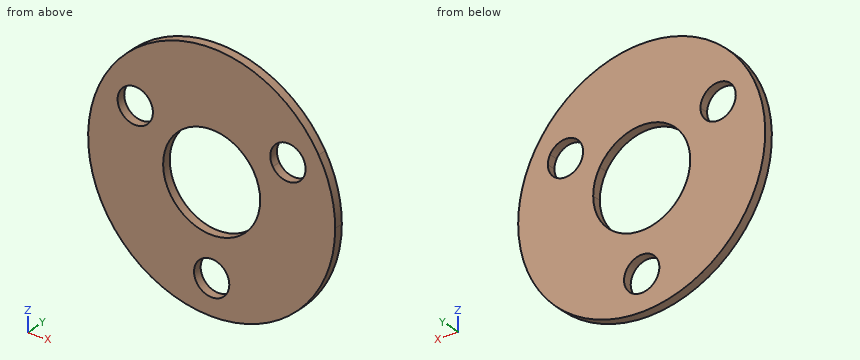
```python
from build123d import *

# Parameters (mm, degrees)
F0_R     = 12.7
F1_DEPTH = 6.35


with BuildPart() as f1:
    # F0 (on Front) → F1 (new body)
    with BuildSketch(Plane.XZ):
        with BuildLine():
            Line((43.995441, 25.40078), (30.245937, 17.4625))
            ThreePointArc((30.245937, 17.4625), (33.734959, 9.039255), (34.925, 0))
            ThreePointArc((34.925, 0), (-9.039255, -33.734959), (-30.245937, 17.4625))
            Line((-30.245937, 17.4625), (-43.994091, 25.4))
            ThreePointArc((-43.994091, 25.4), (-61.342613, 20.751477), (-65.991136, 38.1))
            Line((-65.991136, 38.1), (-76.989658, 44.45))
            ThreePointArc((-76.989658, 44.45), (-23.009013, -85.870806), (88.9, 0))
            ThreePointArc((88.9, 0), (85.870806, 23.009013), (76.989658, 44.45))
            Line((76.989658, 44.45), (65.98911, 38.09883))
            ThreePointArc((65.98911, 38.09883), (67.176599, 35.121917), (67.581014, 31.942516))
            ThreePointArc((67.581014, 31.942516), (58.275364, 19.704527), (43.995441, 25.40078))
        make_face()
        with Locations((0, -63.5)):
            Circle(F0_R, mode=Mode.SUBTRACT)
        with BuildLine():
            ThreePointArc((-30.245937, 17.4625), (0, 34.925), (30.245937, 17.4625))
            Line((30.245937, 17.4625), (43.995441, 25.40078))
            ThreePointArc((43.995441, 25.40078), (48.531014, 42.941039), (65.98911, 38.09883))
            Line((65.98911, 38.09883), (76.989658, 44.45))
            ThreePointArc((76.989658, 44.45), (0, 88.9), (-76.989658, 44.45))
            Line((-76.989658, 44.45), (-65.991136, 38.1))
            ThreePointArc((-65.991136, 38.1), (-51.705611, 44.017258), (-42.292613, 31.75))
            ThreePointArc((-42.292613, 31.75), (-42.725355, 28.462998), (-43.994091, 25.4))
            Line((-43.994091, 25.4), (-30.245937, 17.4625))
        make_face()
    extrude(amount=F1_DEPTH)


solid = f1.part
```
Model file for the job. Use its own axes, mm. Coordinates: 2 decimals unless noted, no trailing zeros. Order: outer loops, then holes, each group sorted by start corner. A loop starts at its lowest first (then second) coordinate and runs counter-clockwise, first axis right, second up. Notation, with made-up numbers: (0.5, -23.75) - (36.5, -23.75) arc R33 cw to (36.5, 8.25) - close; hole circle Ø10 at (19, 11.5). An arc over 180 degrees is marked (long way). Return JSON: item names as keys, results as strings. Group by question number.
1) Flat gauge pins, fed straight in: P1, Ø1, axis at y = -5.5, z = -41.5, coming from the -X side; P2, Ø1, axis at y = -5.5, z = -48, coming from the +X side; P3, Ø3, axis at x = 62.5, y = -0.5, coming from the -Z side. Where does each tip first touch, or does it go through?
2) Saw through at B-B, the plane y = -4.5. Count the separate pieces of the cut face and the enclosed holes in it, plus the area to 3 significant figures.
3) Probe line 1 (X direction, y = -3.5, z = 0) (3 decimals); line 2 (X direction, y = -2, z = 35.5); line 3 (Z direction, x = 30.5, y = -6). List the from-to ranges inside material, lowest first. Write a range as from..to.
4) Saw through at C-C, the plane z = -63.5. Write the cut outline in (x, y).
5) Saw through at A-A, the plane x = 0. Write the cut outline in (y, z) (3 decimals), plus the area to 3 significant figures.
6) Saw through at D-D, the plane x = -19. Write the cut outline in (y, z), plus the area to 3 significant figures.
Values found:
{
 "1": {"P1": "stops at x = -78.88", "P2": "stops at x = 75.15", "P3": "stops at z = -64.67"},
 "2": {"separate pieces": "1", "enclosed holes": "4", "area": "19,500 mm²"},
 "3": {"line 1": "x = -88.9..-34.925, 34.925..88.9", "line 2": "x = -81.5..-67.13, -42.86..42.69, 67.07..81.5", "line 3": "z = -83.5..-17.01, 17.01..83.5"},
 "4": {"outline": "(-62.22, -6.35) - (-12.7, -6.35) - (-12.7, 0) - (-62.22, 0) - close; (12.7, -6.35) - (62.22, -6.35) - (62.22, 0) - (12.7, 0) - close"},
 "5": {"outline": "(-6.35, -88.9) - (0, -88.9) - (0, -76.2) - (-6.35, -76.2) - close; (-6.35, -50.8) - (0, -50.8) - (0, -34.925) - (-6.35, -34.925) - close; (-6.35, 34.925) - (0, 34.925) - (0, 88.9) - (-6.35, 88.9) - close", "area": "524 mm²"},
 "6": {"outline": "(-6.35, -86.85) - (0, -86.85) - (0, -29.3) - (-6.35, -29.3) - close; (-6.35, 29.3) - (0, 29.3) - (0, 86.85) - (-6.35, 86.85) - close", "area": "731 mm²"}
}
